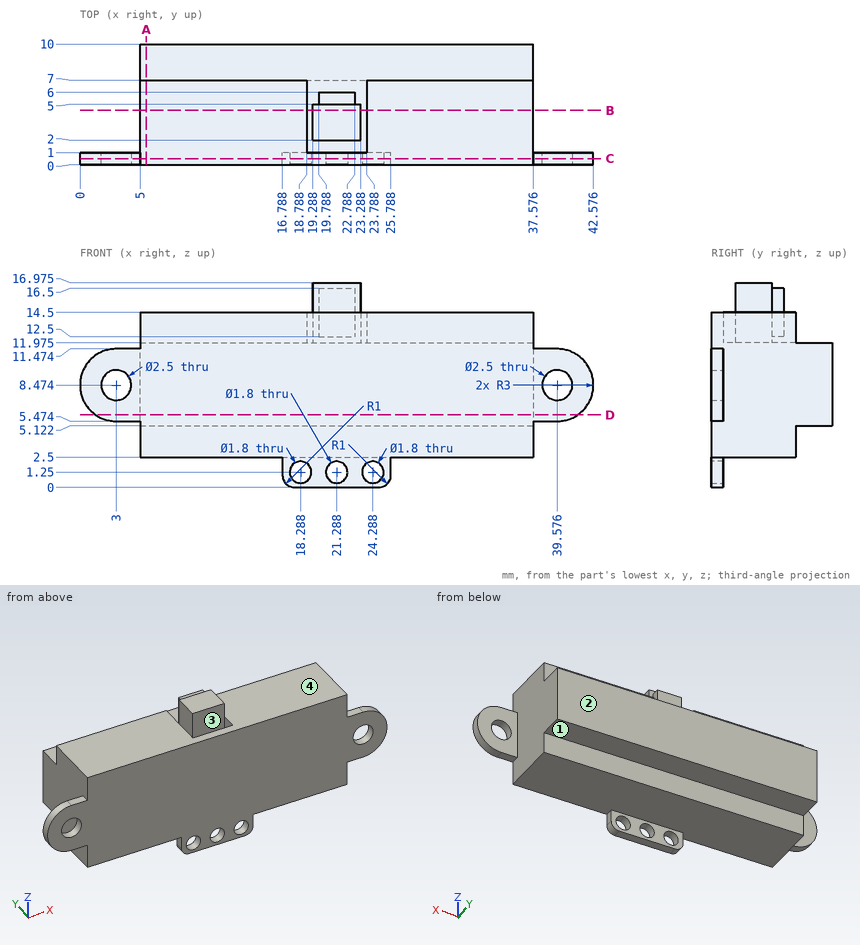
Verification items for this drawing (mm, ordinates from the low corner). A direction names the side the tool comes from. Round coordinates to 2 decimals unless told otherwise and drop trailing zeros. Loops run counter-clockwise (first coordinate to the right, second up) from the corner with the lowest first, then second, coordinate; pieces in that order, holes last. Notation, with made-up numbers: (-9, -12) -> (11, -12) arc R21 ccw to (11, 16) -> close; hole circle Ø5 at (-26.75, -2). An arc over 180 degrees is marked (long way). Answer in a Markdown table with one row per item.
Q1. Sectioned sample at D-D on z = 6. Enter the section's corners in (x, y), then the cut area to 3 significant figures.
Data:
| item | result |
|---|---|
| outline | (1.3, 0) -> (41.27, 0) -> (41.27, 1) -> (37.58, 1) -> (37.58, 10) -> (5, 10) -> (5, 1) -> (1.3, 1) -> close |
| area | 333 mm^2 |
Q2. Thickness scan on L1, parallel to X at y = 0.55, z = 1.25; L2, parallel to X at y = 8, z = 10.75; L3, parallel to Z at x = 13.5, y = 0.5. Record the ranges inside material, lowest first.
Data:
| item | result |
|---|---|
| L1 | x = 16.79 to 17.39, 19.19 to 20.39, 22.19 to 23.39, 25.19 to 25.79 |
| L2 | x = 5 to 37.58 |
| L3 | z = 2.5 to 14.5 |
Q3. Release check for a two-part mould opening along X. For the marked faces 3 and 4 record: released by +X, released by -X, zero draft, split by the parting line, or undercut.
Data:
| item | result |
|---|---|
| face 3 | undercut |
| face 4 | zero draft |
Q4. Sectioned sample at C-C on y = 0.5. Enter the section's corners in (x, z), then the cut area to 3 significant figures.
Data:
| item | result |
|---|---|
| outline | (3, 5.47) -> (5, 5.47) -> (5, 2.5) -> (16.79, 2.5) -> (16.79, 1) arc R1 ccw to (17.79, 0) -> (24.79, 0) arc R1 ccw to (25.79, 1) -> (25.79, 2.5) -> (37.58, 2.5) -> (37.58, 5.47) -> (39.58, 5.47) arc R3 ccw to (39.58, 11.47) -> (37.58, 11.47) -> (37.58, 14.5) -> (5, 14.5) -> (5, 11.47) -> (3, 11.47) arc R3 ccw to start; hole circle Ø2.5 at (3, 8.47); hole circle Ø1.8 at (18.29, 1.25); hole circle Ø1.8 at (21.29, 1.25); hole circle Ø1.8 at (24.29, 1.25); hole circle Ø2.5 at (39.58, 8.47) |
| area | 448 mm^2 |
Q5. Sectioned sample at B-B on y = 4.5. Enter the section's corners in (x, z) (1 decimal).
Data:
| item | result |
|---|---|
| outline | (5, 2.5) -> (37.6, 2.5) -> (37.6, 14.5) -> (23.8, 14.5) -> (23.8, 12) -> (23.3, 12) -> (23.3, 17) -> (19.3, 17) -> (19.3, 12) -> (18.8, 12) -> (18.8, 14.5) -> (5, 14.5) -> close |
Q6. Sectioned sample at A-A on x = 5.5. Enter the section's corners in (y, z) (1 decimal), then the cut area to 3 significant figures.
Data:
| item | result |
|---|---|
| outline | (0, 2.5) -> (7, 2.5) -> (7, 5.1) -> (10, 5.1) -> (10, 12) -> (7, 12) -> (7, 14.5) -> (0, 14.5) -> close |
| area | 105 mm^2 |
Q7. Go/stop test with flat-tipped pins: P1, Ø10, axis at x = 21.5, z = 15, coming from the -Y side; P2, Ø1.5, axis at y = 3.5, z = 15, coming from the -X side; P3, Ø0.8, axis at x = 20.5, y = 5.5, coming from the +Z side; P4, Ø0.8, axis at x = 4.5, y = 0.5, coming from the -Z side. Record where each tip stops, or that it passes through.
Data:
| item | result |
|---|---|
| P1 | stops at y = 0 |
| P2 | stops at x = 5 |
| P3 | stops at z = 16.5 |
| P4 | stops at z = 5.47 |
Q8. Set-up check for the marked faces 1 and 2: record each of +Z, -Z, +X, -X, +Y, -Y from which the full face is reachable in a straight line by a thin tool's end or side.
Data:
| item | result |
|---|---|
| face 1 | -Z, +X, -X, +Y |
| face 2 | +Z, -Z, +X, -X, +Y |
